Read the model definition and answer for the solid it produces. Units are mm, in the model's axes. A direction names the side the tool comes from. Give positions to 0.01 mm unless a question says otherwise; leave off trailing zeros. Loops run counter-clockwise (first coordinate to the right, second up) from the corner with the lowest first, then second, coordinate; pieces in that order, holes last. Notation, with made-up numbers: (-36.75, 62) -> (11.25, 62) arc R27 ccw to (11.25, 84) -> close; hole circle Ø8 at (-1.5, -27). An arc over 180 degrees is marked (long way). Write each question's results on one line, items separated by ' | '. Start each with the question number.
Item 1: Which of the six approach directions +Z, -Z, +X, -X, +Y, -Y give full straight-line access (tool end or side, diameter ignored) to faces 4 (the flat face through (17.3, 0, 21)), 5 (the flat face through (0, 2, -31.069))?
Item 2: Determine the mould class of faces 1 (the flat face through (0, 3, -31.814)), 2 (the flat face through (-1, 2, -30)), 3 (the flat face through (17.3, 5, 21)) for opening direction Z: +Z half, -Z half, draft (parallel to the pull), parting line (faces both ways), or undercut.
Item 3: Find the intervals of material crossed by line 1 (X direction, y = 4, z = 0); line 2 (X direction, y = 3.7, z = 6); line 3 (Z direction, x = -14.5, y = 3.1), in increasing order.
Item 4: Each of these flat-tipped pins is pushed along its axis until it touches: P1, Ø1.4, axis at y = 3, z = -30.5, coming from the +X side; P2, Ø1, axis at y = 3, z = -30.5, coming from the -X side; P3, Ø1.5, axis at x = -2, y = 2.5, coming from the +Z side. Where does it stop, or does it pass through?
Item 5: Section C-C on x = 22 is taken. Write down the section's boundary in (y, z), and give its area (3 significant figures).
Item 6: Section B-B on y = 1.15 is taken. Write down the section's boundary in (x, z).
Item 7: Section A-A on z = -6 is taken. Write down the section's boundary in (x, y), and give its area (3 significant figures).
```python
from build123d import *

# Parameters (mm, degrees)
ESBO_O1_R                = 29
ESBO_O1_R_2              = 27
RESSALTO_EXTRUS_O1_DEPTH = 5
ESBO_O2_W                = 4
ESBO_O2_H                = 4
RESSALTO_EXTRUS_O2_DEPTH = 5
FILETE1_R                = 1
ESBO_O3_W                = 2
ESBO_O3_H                = 1.302391812
CORTE_EXTRUS_O1_DEPTH    = 44.337755413


with BuildPart() as part:
    # Esboço1 → Ressalto-extrusão1 (new body)
    with BuildSketch(Plane(origin=(0, 0, 0), x_dir=(1, 0, 0), z_dir=(0, 1, 0))):
        with Locations(Location((0, 0, 0), (0, 0, 270))):
            Circle(ESBO_O1_R)
        with Locations(Location((0, 0, 0), (0, 0, 270))):
            Circle(ESBO_O1_R_2, mode=Mode.SUBTRACT)
    extrude(amount=RESSALTO_EXTRUS_O1_DEPTH)

    # Esboço2 → Ressalto-extrusão2 (add, through all)
    with BuildSketch(Plane(origin=(0, 5, 0), x_dir=(1, 0, 0), z_dir=(0, 1, 0))):
        with Locations((0, 29.814478531)):
            Rectangle(ESBO_O2_W, ESBO_O2_H)
    extrude(amount=-RESSALTO_EXTRUS_O2_DEPTH)

    # Filete1
    filete1_edges = [part.edges().sort_by_distance(p)[0] for p in [
        (-2, 2.5, -28.930952283),
        (2, 2.5, -28.930952283),
        (2, 2.5, -31.814478531),
        (-2, 2.5, -31.814478531),
    ]]
    fillet(filete1_edges, radius=FILETE1_R)

    # Esboço3 → Corte-extrusão1 (cut, through all)
    with BuildSketch(Plane.XZ):
        with Locations((0, -30.417415502)):
            Rectangle(ESBO_O3_W, ESBO_O3_H)
    extrude(amount=-CORTE_EXTRUS_O1_DEPTH, mode=Mode.SUBTRACT)


solid = part.part
```
Findings:
1) face 4: +Z, -Z, +X, -X, -Y | face 5: +Y, -Y
2) face 1: -Z half | face 2: undercut | face 3: draft
3) line 1: -29 to -27, 27 to 29 | line 2: -28.37 to -26.32, 26.32 to 28.37 | line 3: -25.11 to -22.78, 22.78 to 25.11
4) P1: x = 2 | P2: x = -2 | P3: z = 28.97
5) outline: (0, -18.89) -> (5, -18.89) -> (5, -15.65) -> (0, -15.65) -> close; (0, 15.65) -> (5, 15.65) -> (5, 18.89) -> (0, 18.89) -> close | area: 32.4 mm2
6) outline: (-2.9, -28.85) arc R1 cw to (-2, -29.85) -> (-2, -30.81) arc R1 ccw to (-1, -31.81) -> (1, -31.81) arc R1 ccw to (2, -30.81) -> (2, -29.85) arc R1 cw to (2.9, -28.85) arc R29 ccw (long way) to start; hole circle Ø54 at (0, 0); hole (-1, -31.07) -> (1, -31.07) -> (1, -29.77) -> (-1, -29.77) -> close
7) outline: (-28.37, 0) -> (-26.32, 0) -> (-26.32, 5) -> (-28.37, 5) -> close; (26.32, 0) -> (28.37, 0) -> (28.37, 5) -> (26.32, 5) -> close | area: 20.5 mm2
